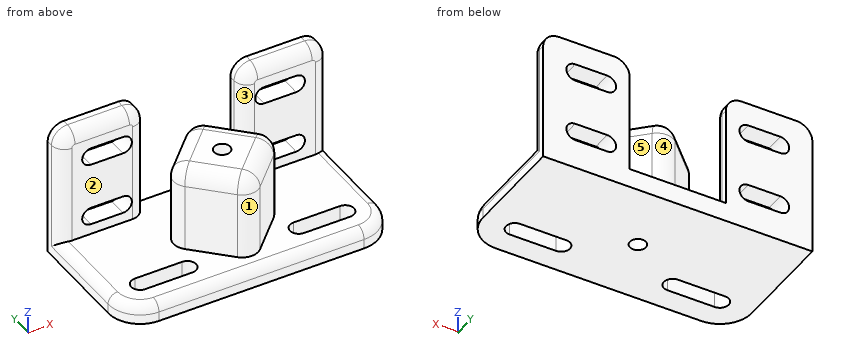
from build123d import *

# Parameters (mm, degrees)
F1_DEPTH = 6
F0_R     = 2.5
F2_DEPTH = 32
F3_R     = 5
F4_R     = 3
F6_DEPTH = 6
F7_R     = 4


with BuildPart() as f1:
    # F0 (on Top) → F1 (new body)
    with BuildSketch(Plane.XY):
        with BuildLine():
            Line((84, 0), (0, 0))
            Line((0, 0), (0, -32))
            ThreePointArc((0, -32), (2.928932, -39.071068), (10, -42))
            Line((10, -42), (74, -42))
            ThreePointArc((74, -42), (81.071068, -39.071068), (84, -32))
            Line((84, -32), (84, 0))
        make_face()
        with BuildLine():
            ThreePointArc((10, -34.75), (7.25, -32), (10, -29.25))
            Line((10, -29.25), (24.74713, -29.25))
            ThreePointArc((24.74713, -29.25), (27.49713, -32), (24.74713, -34.75))
            Line((24.74713, -34.75), (10, -34.75))
        make_face(mode=Mode.SUBTRACT)
        with BuildLine():
            ThreePointArc((59.536784, -34.75), (56.786784, -32), (59.536784, -29.25))
            Line((59.536784, -29.25), (74, -29.25))
            ThreePointArc((74, -29.25), (76.75, -32), (74, -34.75))
            Line((74, -34.75), (59.536784, -34.75))
        make_face(mode=Mode.SUBTRACT)
        Polygon((42.141957, -3.74713), (59.536784, -21.141957), (42.141957, -38.536784), (24.74713, -21.141957), align=None, mode=Mode.SUBTRACT)
    extrude(amount=F1_DEPTH)

    # F0 (on Top) → F2 (join)
    with BuildSketch(Plane.XY):
        Polygon((42.141957, -38.536784), (59.536784, -21.141957), (42.141957, -3.74713), (24.74713, -21.141957), align=None)
        with Locations((42.00013, -21.141957)):
            Circle(F0_R, mode=Mode.SUBTRACT)
    extrude(amount=F2_DEPTH)

    # F3
    f3_edges = [f1.edges().sort_by_distance(p)[0] for p in [
        (42.141957, -38.536784, 19),
        (24.74713, -21.141957, 19),
        (59.536784, -21.141957, 19),
        (42.141957, -3.74713, 19),
        (33.444544, -12.444544, 32),
        (50.83937, -12.444544, 32),
        (50.83937, -29.83937, 32),
        (33.444544, -29.83937, 32),
    ]]
    fillet(f3_edges, radius=F3_R)

    # F4
    f4_edges = [f1.edges().sort_by_distance(p)[0] for p in [
        (42, -42, 6),
    ]]
    fillet(f4_edges, radius=F4_R)

    # F5 (on Front) → F6 (join)
    with BuildSketch(Plane.XZ):
        with BuildLine():
            Line((0, 37), (0, 0))
            Line((0, 0), (27, 0))
            Line((27, 0), (27, 37))
            ThreePointArc((27, 37), (25.535534, 40.535534), (22, 42))
            Line((22, 42), (5, 42))
            ThreePointArc((5, 42), (1.464466, 40.535534), (0, 37))
        make_face()
        with BuildLine():
            ThreePointArc((10, 9.25), (7.25, 12), (10, 14.75))
            Line((10, 14.75), (20, 14.75))
            ThreePointArc((20, 14.75), (22.75, 12), (20, 9.25))
            Line((20, 9.25), (10, 9.25))
        make_face(mode=Mode.SUBTRACT)
        with BuildLine():
            ThreePointArc((20, 34.75), (22.75, 32), (20, 29.25))
            Line((20, 29.25), (10, 29.25))
            ThreePointArc((10, 29.25), (7.25, 32), (10, 34.75))
            Line((10, 34.75), (20, 34.75))
        make_face(mode=Mode.SUBTRACT)
        with BuildLine():
            Line((84, 0), (84, 37))
            ThreePointArc((84, 37), (82.535534, 40.535534), (79, 42))
            Line((79, 42), (62, 42))
            ThreePointArc((62, 42), (58.464466, 40.535534), (57, 37))
            Line((57, 37), (57, 0))
            Line((57, 0), (84, 0))
        make_face()
        with BuildLine():
            ThreePointArc((64, 9.25), (61.25, 12), (64, 14.75))
            Line((64, 14.75), (74, 14.75))
            ThreePointArc((74, 14.75), (76.75, 12), (74, 9.25))
            Line((74, 9.25), (64, 9.25))
        make_face(mode=Mode.SUBTRACT)
        with BuildLine():
            ThreePointArc((64, 29.25), (61.25, 32), (64, 34.75))
            Line((64, 34.75), (74, 34.75))
            ThreePointArc((74, 34.75), (76.75, 32), (74, 29.25))
            Line((74, 29.25), (64, 29.25))
        make_face(mode=Mode.SUBTRACT)
    extrude(amount=F6_DEPTH)

    # F7
    f7_edges = [f1.edges().sort_by_distance(p)[0] for p in [
        (0, -6, 20),
        (84, -6, 20),
    ]]
    fillet(f7_edges, radius=F7_R)


solid = f1.part
CAD build for the part. Positions are in the model's coordinates, mm. Face numbers are marked on the shaded views. A direction names the side the tool comes from. Give positions to 0.01 mm unless a question says otherwise; leave off trailing zeros. Write each loop counter-clockwise with the first axis right and the second up, starting at its lowest first coordinate (ties: lowest second). Pieces come first, ordered by that corner, then holes. Notation, with made-up numbers: (-10.5, 3.25) -> (8.5, 3.25) arc R15 cw to (8.5, 21.25) -> close; hole circle Ø6 at (-24, 61). An arc over 180 degrees is marked (long way). Return JSON: item names as keys, results as strings.
Item 1: Band-saw the part on A-A (z = 26). List the corners of the cut face in (x, y).
Answer below:
{"outline": "(0, -2) arc R4 ccw to (4, -6) -> (23, -6) arc R4 ccw to (27, -2) -> (27, 0) -> (0, 0) -> close; (28.28, -24.68) -> (38.61, -35) arc R5 ccw to (45.68, -35) -> (56, -24.68) arc R5 ccw to (56, -17.61) -> (45.68, -7.28) arc R5 ccw to (38.61, -7.28) -> (28.28, -17.61) arc R5 ccw to start; (57, -2) arc R4 ccw to (61, -6) -> (80, -6) arc R4 ccw to (84, -2) -> (84, 0) -> (57, 0) -> close; hole circle Ø5 at (42, -21.14)"}
Item 2: Drill centre lines: probe 1 along X at (y, z) = (-32.5, 5); probe 2 along Y at (x, z) = (80, 34); probe 3 along Z at (x, y) = (76, -29). Where is each one in solid material? Low to high.
Answer below:
{"probe 1": "x = 0.78 to 7.3, 27.45 to 56.83, 76.7 to 83.22", "probe 2": "y = -6 to 0", "probe 3": "z = 0 to 6"}
Item 3: Tool access for the marked faces 1, 2, 3, 4 and 5: list every direction of +Z, -Z, +X, -X, +Y, -Y with a clear straight run to the whole face (end or side of a thin tool).
Answer below:
{"face 1": "+Z, -Y", "face 2": "+Z, -X, -Y", "face 3": "+Z", "face 4": "+Z, +Y", "face 5": "+Z, +X, +Y"}
Item 4: Drop flat-ended pins along their axis: pin 1 (1 mm diameter, centred on y = -14.5, z = 27.5, fed in from +X); pin 2 (10 mm diameter, centred on y = -37.5, z = 19.5, fed in from +X); pin 3 (4 mm diameter, centred on x = 10.5, y = -27, fed in from +Z). Give the stop position or say it passes through.
Answer below:
{"pin 1": "stops at x = 53.36", "pin 2": "stops at x = 48.18", "pin 3": "stops at z = 6"}
Item 5: Band-saw the part on B-B (z = 12). Give the number of separate pieces and of enclosed holes in the cut face, then the cut area to 3 significant figures.
Answer below:
{"separate pieces": "5", "enclosed holes": "1", "area": "688 mm2"}
